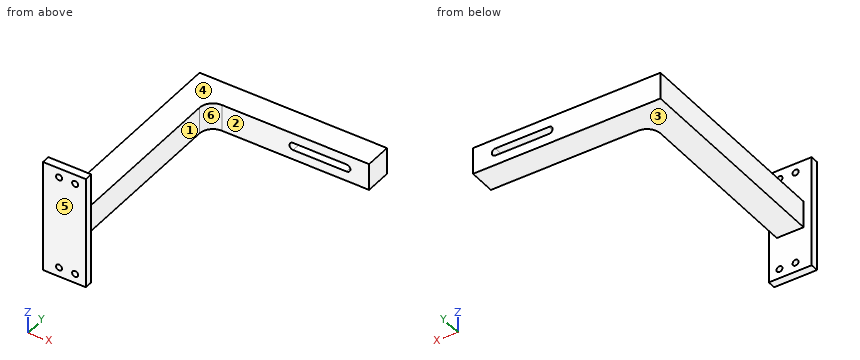
```python
from build123d import *

# Parameters (mm, degrees)
SKETCH2_W                       = 32
SKETCH2_H                       = 84
STALK_FLANGE_32X84X6_DEPTH      = 6
F_4_5_4_5_DIAMETER_HOLE1_D      = 4.5
SKETCH5_W                       = 20
SKETCH5_H                       = 20
VERTICAL_COLUMN_20X20X160_DEPTH = 160
SKETCH6_W                       = 120
SKETCH6_H                       = 20
HORIZONTAL_ARM_20X20X120_DEPTH  = 10
INSIDE_FILLET_R10_R             = 10
TIP_SLOT_40X5_5_THRU_DEPTH      = 259.758574737


with BuildPart() as part:
    # Sketch2 → Stalk_Flange_32x84x6 (new body)
    with BuildSketch(Plane(origin=(0, 0, 0), x_dir=(1, 0, 0), z_dir=(0, 1, 0))):
        with Locations((64, 0)):
            Rectangle(SKETCH2_W, SKETCH2_H)
    extrude(amount=STALK_FLANGE_32X84X6_DEPTH)

    # Ø4.5 (4.5) Diameter Hole1 (through all)
    with Locations(Plane(origin=(0, 6, 0), x_dir=(1, 0, 0), z_dir=(0, 1, 0))):
        with Locations((60, 35), (72, 35), (60, -35), (72, -35)):
            Hole(F_4_5_4_5_DIAMETER_HOLE1_D / 2)

    # Sketch5 → Vertical_Column_20x20x160 (add)
    with BuildSketch(Plane(origin=(0, 6, 0), x_dir=(1, 0, 0), z_dir=(0, 1, 0))):
        with Locations((64, 0)):
            Rectangle(SKETCH5_W, SKETCH5_H)
    extrude(amount=VERTICAL_COLUMN_20X20X160_DEPTH)

    # Sketch6 → Horizontal_Arm_20x20x120 (add, symmetric)
    with BuildSketch(Plane.XY):
        with Locations((134, 156)):
            Rectangle(SKETCH6_W, SKETCH6_H)
    extrude(amount=HORIZONTAL_ARM_20X20X120_DEPTH, both=True)

    # Inside_Fillet_R10
    inside_fillet_r10_edges = [part.edges().sort_by_distance(p)[0] for p in [
        (74, 146, 0),
    ]]
    fillet(inside_fillet_r10_edges, radius=INSIDE_FILLET_R10_R)

    # Sketch7 → Tip_Slot_40x5.5_THRU (cut, through all)
    with BuildSketch(Plane(origin=(0, 166, 0), x_dir=(1, 0, 0), z_dir=(0, 1, 0))):
        with BuildLine():
            Line((177.25, -2.75), (137.25, -2.75))
            ThreePointArc((137.25, -2.75), (134.5, 0), (137.25, 2.75))
            Line((137.25, 2.75), (177.25, 2.75))
            ThreePointArc((177.25, 2.75), (180, 0), (177.25, -2.75))
        make_face()
    extrude(amount=-TIP_SLOT_40X5_5_THRU_DEPTH, mode=Mode.SUBTRACT)


solid = part.part
```
Design review of the part built by this model. Coordinates are the model's own, in mm. Face numbers are marked on the shaded views. A direction names the side the tool comes from. Give positions to 0.01 mm unless a question says otherwise; leave off trailing zeros. Loops run counter-clockwise (first coordinate to the right, second up) from the corner with the lowest first, then second, coordinate; pieces in that order, holes last. Notation, with made-up numbers: M 10.5,86 L 65.5,86 A29 cw 65.5,110 Z; hole C -34.5,2 d11. An arc over 180 degrees is marked long. Return JSON: item names as keys, results as strings. Group by question number.
Item 1: Insertion check: pin 1 Ø1.8 at (y, z) = (2.5, -0.5) entering from +X; pin 2 Ø6 at (x, y) = (158, 154) entering from -Z; pin 3 Ø6 at (x, z) = (72, 35) entering from +Y. Each pin has a flat end and moves straight along its axis. Give the tip position at first contact, or say it passes through.
Item 2: We need section A-A (z = 0). Give the boundary of the cut face in (x, y).
Item 3: Tool access review of the marked faces 1, 2 and 3: name each direction out of +Z, -Z, +X, -X, +Y, -Y from which nothing blocks a thin tool from reaching the whole face with its end or side.
Item 4: We need section B-B (x = 60). Give the boundary of the cut face in (y, z), and give its area (3 significant figures).
Item 5: We need section C-C (z = 35). Give the boundary of the cut face in (x, y).
Item 6: For probe 1 along X at (y, z) = (2, 35); probe 2 along Z at (x, y) = (72, 3); probe 3 along Y at (x, z) = (177, -3), list the stretches that pass through material, from the lowest coordinate up.
Item 7: Mouldability with a two-part tool opening along Y and no side actions: class the marked faces 4, 5 and 6 as released by +Y, released by -Y, zero draft, split by the parting line, or undercut.
Item 8: We need section D-D (y = 109). Give the boundary of the cut face in (x, z).
Output:
{
 "1": {"pin 1": "stops at x = 80", "pin 2": "stops at z = -10", "pin 3": "stops at y = 6"},
 "2": {"outline": "M 48,0 L 80,0 L 80,6 L 74,6 L 74,136 A10 cw 84,146 L 134.5,146 L 134.5,166 L 54,166 L 54,6 L 48,6 Z; M 180,146 L 194,146 L 194,166 L 180,166 Z"},
 "3": {"face 1": "+Z, -Z, +X", "face 2": "+Z, -Z, +X, -Y", "face 3": "-Z, +X, -X, +Y"},
 "4": {"outline": "M 0,-42 L 6,-42 L 6,-37.25 L 0,-37.25 Z; M 0,-32.75 L 6,-32.75 L 6,-10 L 166,-10 L 166,10 L 6,10 L 6,32.75 L 0,32.75 Z; M 0,37.25 L 6,37.25 L 6,42 L 0,42 Z", "area": "3,650 mm^2"},
 "5": {"outline": "M 48,0 L 57.75,0 L 57.75,6 L 48,6 Z; M 62.25,0 L 69.75,0 L 69.75,6 L 62.25,6 Z; M 74.25,0 L 80,0 L 80,6 L 74.25,6 Z"},
 "6": {"probe 1": "x = 48 to 57.75, 62.25 to 69.75, 74.25 to 80", "probe 2": "z = -42 to -37.25, -32.75 to 32.75, 37.25 to 42", "probe 3": "y = 146 to 166"},
 "7": {"face 4": "zero draft", "face 5": "released by -Y", "face 6": "undercut"},
 "8": {"outline": "M 54,-10 L 74,-10 L 74,10 L 54,10 Z"}
}
